Autodesk Fusion 360 part; units mm, degrees
sketch "Sketch1" plane through (0, 0, 0) normal (0, 0, 1) x (1, 0, 0)
  line L0 (0, -5) -> (22, -5)
  arc A0 (22, -5) -> (22, 5) centre (22, 0) ccw
  line L1 (22, 5) -> (0, 5)
  arc A1 (0, 5) -> (0, -5) centre (0, 0) ccw
  line L2 (0, 0) -> (22, 0) construction
  circle A2 centre (0, 0) radius 1.5
  line L3 (20.05, 5) -> (60.7446, 21.7316)
  line L4 (60.7446, 21.7316) -> (64.6864, 12.1444)
  line L5 (64.6864, 12.1444) -> (23.9013, -4.6244)
  line L6 (50.6615, 17.5859) -> (62.7155, 16.938)
  line L7 (48.8067, 5.6155) -> (42.5976, 7.9233)
  line L8 (42.5976, 7.9233) -> (26.963, 0.6072)
  circle A3 centre (22, 0) radius 1.5
  dimension "d1" = 22
  dimension "d2" = 5
  dimension "d3" = 3
  dimension "d4" = 157.65
  dimension "d5" = 44
  dimension "d6" = 1.95
  dimension "d7" = 3
extrude "Extrude1" add sketch "Sketch1" along normal blind 3 contours L0 A0 L1 A1 | A0 L1 L3 L4 L5 L6 L7 L8
sketch "Sketch2" plane through (0, 0, 0) normal (0, 0, 1) x (1, 0, 0)
  circle A0 centre (14, 12) radius 3.5
  circle A1 centre (14, 12) radius 1.5
  circle A2 centre (45, 12) radius 1.5
  circle A3 centre (45, 12) radius 3.5
  line L0 (14, 12) -> (45, 12)
  line L1 (17.1623, 13.5) -> (41.8377, 13.5)
  line L2 (17.1623, 10.5) -> (41.8377, 10.5)
  dimension "d10" = 3
  dimension "d11" = 3
  dimension "d12" = 7
  dimension "d13" = 7
  dimension "d14" = 31
  dimension "d15" = 1.5
Input: part model. Units: mm. Frame: model coordinates. A direction names the side the tool comes from. Give positions to 0.01 mm unless a question says otherwise; leave off trailing zeros. Loops run counter-clockwise (first coordinate to the right, second up) from the corner with the lowest first, then second, coordinate; pieces in that order, holes last. Notation, with made-up numbers: (88, 47.5) - (125, 47.5) arc R23 ccw to (125, 66.5) - close; hole circle Ø2 at (0, 80.5). An arc over 180 degrees is marked (long way). Use CSV: the item, a comma, the result in double quotes. Start each with the question number.
Item 1: Reachability of faces 5 (the flat face through (45.75, 6.75, 1.48)), 6 (the flat face through (10, 5, 1)), 7 (the flat face through (11, -5, 1)) from +Z, -Z, +X, -X, +Y, -Y: full face, straight path, thin tool, end or side. Return the list, or none.
Item 2: Line query: line 1 (Y direction, x = 0, z = 1.05); line 2 (X direction, y = -0.5, z = 0.55); line 3 (Y direction, x = 22, z = 1.7). Output: solid intervals per line, ascending.
Item 3: Section B-B on y = 7. Return loops of the section in (x, z), then the cut area to 3 significant figures.
Item 4: Section D-D on y = -3. Return loops of the section in (x, z).
Item 5: Section A-A on y = 0. Return loops of the section in (x, z).
Item 6: Mould query, pull axis Y, two halves, no side actions, for faces 1 (the flat face through (35.141, 11.205, 1.479)), 2 (the cylindrical face through (-5, 0, 1)), 3 (the flat face through (30, 6, 0)), 4 (the cylindrical face through (-1.5, -0.07, 1.48)). Classes: pulls with the +Y half, pulls with the -Y half, needs draft (parallel to the pull), parting line crosses it, or undercut.
Item 7: Contact query for flat-ended pins moving along their axis: P1, Ø1.5, axis at y = 7.5, z = 1, coming from the -X side; P2, Ø1.5, axis at x = 6.5, z = 1.5, coming from the +Y side. Output: stop coordinate, or through.
Item 8: Section C-C on z = 1.9. Return loops of the section in (x, y).
Ans:
1,face 5,"+Z, -Z, -Y"
1,face 6,"+Z, -Z, -X, +Y"
1,face 7,"+Z, -Z, +X, -X, -Y"
2,line 1,"y = -5 to -1.5, 1.5 to 5"
2,line 2,"x = -4.97 to -1.41, 1.41 to 20.59, 23.41 to 26.97"
2,line 3,"y = -5 to -1.5, 1.5 to 5.8"
3,outline,"(24.91, 0) - (40.62, 0) - (40.62, 3) - (24.91, 3) - close; (45.08, 0) - (52.17, 0) - (52.17, 3) - (45.08, 3) - close"
3,area,"68.4 mm2"
4,outline,"(-4, 0) - (26, 0) - (26, 3) - (-4, 3) - close"
5,outline,"(-5, 0) - (-1.5, 0) - (-1.5, 3) - (-5, 3) - close; (1.5, 0) - (20.5, 0) - (20.5, 3) - (1.5, 3) - close; (23.5, 0) - (27, 0) - (27, 3) - (23.5, 3) - close"
6,face 1,"pulls with the +Y half"
6,face 2,"parting line crosses it"
6,face 3,"needs draft"
6,face 4,"undercut"
7,P1,"stops at x = 24.31"
7,P2,"stops at y = 5"
8,outline,"(0, -5) - (22, -5) arc R5 ccw to (26.96, 0.61) - (42.6, 7.92) - (48.81, 5.62) - (64.69, 12.14) - (62.72, 16.94) - (50.66, 17.59) - (20.05, 5) - (0, 5) arc R5 ccw to start; hole circle Ø3 at (0, 0); hole circle Ø3 at (22, 0)"
